```python
from build123d import *

# Parameters (mm, degrees)
CHAMFER1_SIZE = 5
CHAMFER2_SIZE = 2
FILLET1_R     = 2.5


with BuildPart() as part:
    # Sketch1 → Revolve1 (revolve)
    with BuildSketch(Plane.XY, mode=Mode.PRIVATE) as revolve1_sk:
        Polygon((0, 0), (0, 29), (60, 29), (60, 50), (100, 50), (100, 35), (210, 35), (210, 0), align=None)
    revolve(revolve1_sk.sketch.rotate(Axis((0, 0, 0), (1, 0, 0)), 90), axis=Axis((0, 0, 0), (1, 0, 0)))

    # Chamfer1
    chamfer1_edges = [part.edges().sort_by_distance(p)[0] for p in [
        (210, 0, -35),
        (0, 0, -29),
    ]]
    chamfer(chamfer1_edges, length=CHAMFER1_SIZE)

    # Chamfer2
    chamfer2_edges = [part.edges().sort_by_distance(p)[0] for p in [
        (100, 0, -50),
        (60, 0, -50),
    ]]
    chamfer(chamfer2_edges, length=CHAMFER2_SIZE)

    # Fillet1
    fillet1_edges = [part.edges().sort_by_distance(p)[0] for p in [
        (100, 0, -35),
        (60, 0, -29),
    ]]
    fillet(fillet1_edges, radius=FILLET1_R)


solid = part.part
```
Input: part model. Units: mm. Frame: model coordinates. A direction names the side the tool comes from. Coordinates: 2 decimals unless noted, no trailing zeros. Order: outer loops, then holes, each group sorted by start corner. A loop starts at its lowest first (then second) coordinate and runs counter-clockwise, first axis right, second up. Notation, with made-up numbers: (31, 25.25) - (73, 25.25) arc R23 ccw to (73, 46.25) - close; hole circle Ø3 at (-35, 26.5). An arc over 180 degrees is marked (long way). Put each result on its own line as item: value.
1. Line query: line 1 along X through (y, z) = (-41.5, 10.5); line 2 along Z through (x, y) = (131, 18); line 3 along Y through (x, z) = (128.5, 1). Output: solid intervals per line, ascending.
Report:
line 1: x = 60 to 100
line 2: z = -30.02 to 30.02
line 3: y = -34.99 to 34.99
2. Reachability of faces 1 (the face through (80.25, -15.02, 47.69)), 2 (the face through (100, 25, -29)), 3 (the face through (31.62, 25.73, 13.38)) from +Z, -Z, +X, -X, +Y, -Y: full face, straight path, thin tool, end or side. Return the list, or none.
Report:
face 1: +X, -X
face 2: +X
face 3: -X
3. Cut plane C-C on x = 111. Return the cut outline in (y, z).
Report:
outline: circle Ø70 at (0, 0)
4. Cut plane A-A on z = 0. Return the cut outline in (x, y).
Report:
outline: (0, -24) - (5, -29) - (57.5, -29) arc R2.5 cw to (60, -31.5) - (60, -48) - (62, -50) - (98, -50) - (100, -48) - (100, -37.5) arc R2.5 cw to (102.5, -35) - (205, -35) - (210, -30) - (210, 30) - (205, 35) - (102.5, 35) arc R2.5 cw to (100, 37.5) - (100, 48) - (98, 50) - (62, 50) - (60, 48) - (60, 31.5) arc R2.5 cw to (57.5, 29) - (5, 29) - (0, 24) - close
5. Contact query for flat-ended pins moving along their axis: pin 1 Ø1 at (y, z) = (24, -26.5) entering from -X; pin 2 Ø4 at (y, z) = (-1.5, -11.5) entering from -X; pin 3 Ø1.5 at (x, y) = (53, 8) entering from -Z; pin 4 Ø8 at (x, z) = (77, -12) entering from -Y. Output: stop coordinate, or through.
Report:
pin 1: stops at x = 60
pin 2: stops at x = 0
pin 3: stops at z = -28.08
pin 4: stops at y = -49.36
